Part print with two shaded views. Sizes in mm from the minimum x, y, z corner. A direction names the side the tool comes from. Give positions to 0.01 mm unless a question says otherwise; leave off trailing zeros. Order: outer loops, then holes, each group sorted by start corner. A loop starts at its lowest first (then second) coordinate and runs counter-clockwise, first axis right, second up. Notation, with made-up numbers: (87.25, 33.5) -> (130.25, 33.5) arc R6 cw to (130.25, 39.5) -> close; hole circle Ø3 at (2.5, 64). An arc over 180 degrees is marked (long way). Answer in a Markdown table with one row per item. Add a question column.
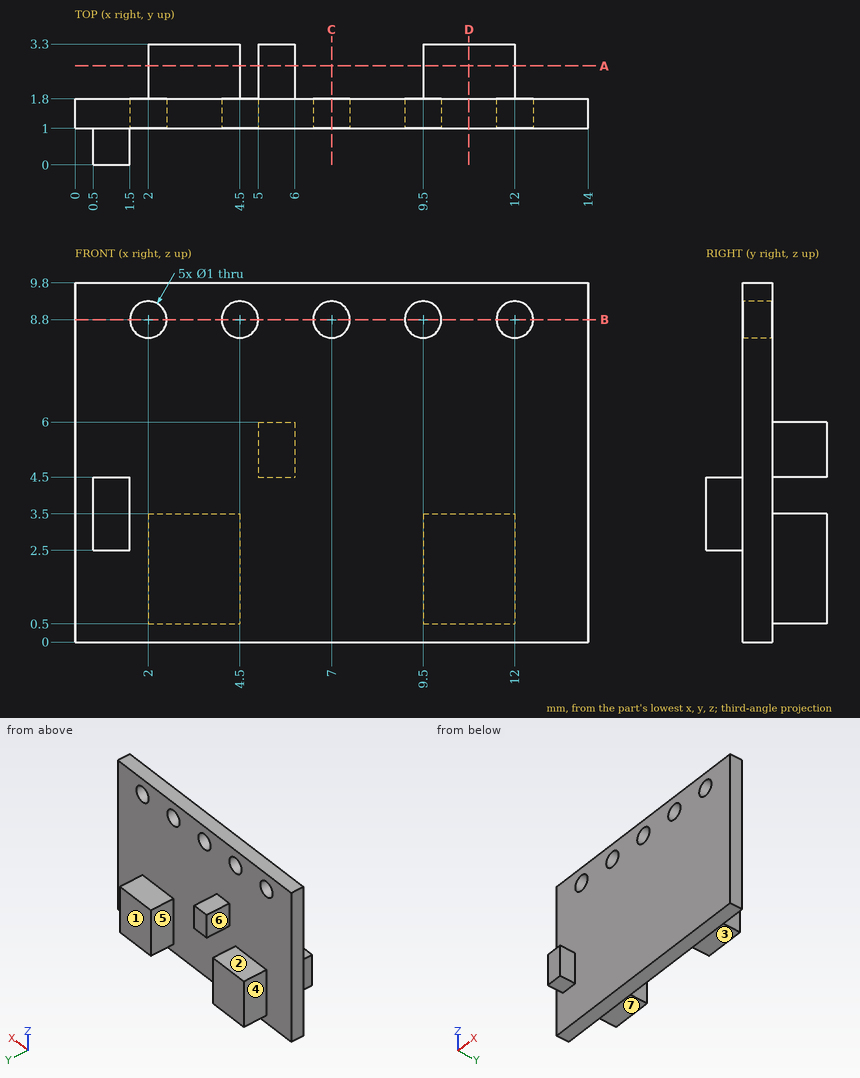
Item 1: Saw through at A-A on y = 2.7. List the corners of the cut face in (x, z), plus the area to 3 significant figures.
Item 2: Pin check, flat tips, straight feed: pin 1 Ø0.8 at (x, y) = (11, 2.5) entering from +Z; pin 2 Ø1.1 at (x, y) = (1, 0.5) entering from +Z; pin 3 Ø0.8 at (y, z) = (2.5, 5) entering from -X; pin 4 Ø1.2 at (y, z) = (3, 2) entering from +X. Stop position of each tip, or through.
Item 3: Saw through at C-C on x = 7. List the corners of the cut face in (y, z).
Item 4: Wall check: line 1 (X direction, y = 1.5, z = 8.8); line 2 (Y direction, x = 5, z = 8); line 3 (X direction, y = 0.65, z = 4). Give the ranges that are in metal, low to high.
Item 5: Two-plate mould, pull along X, no slides. Class the marked faces 5, 6 and 7: pulls with the +X half, pulls with the -X half, needs draft (parallel to the pull), parting line crosses it, or undercut.
Item 6: Saw through at D-D on x = 10.75. List the corners of the cut face in (y, z), plus the area to 3 significant figures.
Item 7: Saw through at B-B on z = 8.8. List the corners of the cut face in (x, y).
Item 8: Which spindle directions (+Z, -Z, +X, -X, +Y, -Y) get a long thin tool onto all of the face, cutting with end or side? Do the marked faces 1, 2, 3 and 4. Say none if no direction does.
Evaluation:
| question | item | result |
|---|---|---|
| 1 | outline | (2, 0.5) -> (4.5, 0.5) -> (4.5, 3.5) -> (2, 3.5) -> close; (5, 4.5) -> (6, 4.5) -> (6, 6) -> (5, 6) -> close; (9.5, 0.5) -> (12, 0.5) -> (12, 3.5) -> (9.5, 3.5) -> close |
| 1 | area | 16.5 mm2 |
| 2 | pin 1 | stops at z = 3.5 |
| 2 | pin 2 | stops at z = 9.8 |
| 2 | pin 3 | stops at x = 5 |
| 2 | pin 4 | stops at x = 12 |
| 3 | outline | (1, 0) -> (1.8, 0) -> (1.8, 8.3) -> (1, 8.3) -> close; (1, 9.3) -> (1.8, 9.3) -> (1.8, 9.8) -> (1, 9.8) -> close |
| 4 | line 1 | x = 0 to 1.5, 2.5 to 4, 5 to 6.5, 7.5 to 9, 10 to 11.5, 12.5 to 14 |
| 4 | line 2 | y = 1 to 1.8 |
| 4 | line 3 | x = 0.5 to 1.5 |
| 5 | face 5 | undercut |
| 5 | face 6 | pulls with the -X half |
| 5 | face 7 | needs draft |
| 6 | outline | (1, 0) -> (1.8, 0) -> (1.8, 0.5) -> (3.3, 0.5) -> (3.3, 3.5) -> (1.8, 3.5) -> (1.8, 9.8) -> (1, 9.8) -> close |
| 6 | area | 12.3 mm2 |
| 7 | outline | (0, 1) -> (1.5, 1) -> (1.5, 1.8) -> (0, 1.8) -> close; (2.5, 1) -> (4, 1) -> (4, 1.8) -> (2.5, 1.8) -> close; (5, 1) -> (6.5, 1) -> (6.5, 1.8) -> (5, 1.8) -> close; (7.5, 1) -> (9, 1) -> (9, 1.8) -> (7.5, 1.8) -> close; (10, 1) -> (11.5, 1) -> (11.5, 1.8) -> (10, 1.8) -> close; (12.5, 1) -> (14, 1) -> (14, 1.8) -> (12.5, 1.8) -> close |
| 8 | face 1 | +Z, -Z, +X, -X, +Y |
| 8 | face 2 | +Z, +X, -X, +Y |
| 8 | face 3 | -Z, +X, -X, +Y |
| 8 | face 4 | +Z, -Z, -X, +Y |
